from build123d import *

# Parameters (mm, degrees)
F0_W         = 126
F0_H         = 10
F0_R         = 1.5
F1_DEPTH     = 8
F2_T1_DEPTH  = 4
F2_T3_DEPTH  = 18
F2_T5_DEPTH  = 129
F2_T7_DEPTH  = 13
F2_S11_W     = 2
F2_S11_H     = 2
F2_T12_DEPTH = 2
F2_S17_W     = 2
F2_S17_H     = 2
F2_T18_DEPTH = 2
F3_T1_DEPTH  = 11
F3_T3_DEPTH  = 4
F3_T5_DEPTH  = 127
F3_S9_W      = 2.04
F3_S9_H      = 2.04
F3_T10_DEPTH = 2.04
F3_S15_W     = 2.04
F3_S15_H     = 2.04
F3_T16_DEPTH = 2.04


# Not quite as in the source:
# - a fillet or chamfer that OpenCascade refuses, or shapes differently, is made with other operations: its cross-section is extruded or revolved along the edge and cut away or added


with BuildPart() as f1:
    # F0 (on Front) → F1 (new body)
    with BuildSketch(Plane.XZ):
        with Locations((0, 5)):
            Rectangle(F0_W, F0_H)
        with Locations((-60, 5)):
            Circle(F0_R, mode=Mode.SUBTRACT)
        with Locations((-40, 5)):
            Circle(F0_R, mode=Mode.SUBTRACT)
        with Locations((60, 5)):
            Circle(F0_R, mode=Mode.SUBTRACT)
    extrude(amount=F1_DEPTH)

    # F2: fillet of radius 2 on 7 edges, made by hand

    # F2_s2 → F2_t1 (cut)
    with BuildSketch(Plane.XZ.offset(2)):
        with BuildLine():
            ThreePointArc((63, 8), (62.4142135624, 9.4142135624), (61, 10))
            Line((61, 10), (63, 10))
            Line((63, 10), (63, 8))
        make_face()
    extrude(amount=F2_T1_DEPTH, mode=Mode.SUBTRACT)

    # F2_s4 → F2_t3 (cut)
    with BuildSketch(Plane.XZ.offset(-5)):
        with BuildLine():
            ThreePointArc((-63, 8), (-62.4142135624, 9.4142135624), (-61, 10))
            Line((-61, 10), (-63, 10))
            Line((-63, 10), (-63, 8))
        make_face()
        with BuildLine():
            ThreePointArc((61, 0), (62.4142135624, 0.5857864376), (63, 2))
            Line((63, 2), (63, 0))
            Line((63, 0), (61, 0))
        make_face()
    extrude(amount=F2_T3_DEPTH, mode=Mode.SUBTRACT)

    # F2_s6 → F2_t5 (cut)
    with BuildSketch(Plane.YZ.offset(-68)):
        with BuildLine():
            ThreePointArc((-2, 10), (-0.5857864376, 9.4142135624), (0, 8))
            Line((0, 8), (0, 10))
            Line((0, 10), (-2, 10))
        make_face()
        with BuildLine():
            ThreePointArc((-6, 10), (-7.4142135624, 9.4142135624), (-8, 8))
            Line((-8, 8), (-8, 10))
            Line((-8, 10), (-6, 10))
        make_face()
    extrude(amount=F2_T5_DEPTH, mode=Mode.SUBTRACT)

    # F2_s8 → F2_t7 (cut)
    with BuildSketch(Plane.XY.offset(-5)):
        with BuildLine():
            ThreePointArc((63, -2), (62.4142135624, -0.5857864376), (61, 0))
            Line((61, 0), (63, 0))
            Line((63, 0), (63, -2))
        make_face()
        with BuildLine():
            ThreePointArc((63, -6), (62.4142135624, -7.4142135624), (61, -8))
            Line((61, -8), (63, -8))
            Line((63, -8), (63, -6))
        make_face()
    extrude(amount=F2_T7_DEPTH, mode=Mode.SUBTRACT)


with BuildPart() as f2_tool10:
    # F2_s11 → F2_t12 (new body)
    with BuildSketch(Plane.YZ.offset(61)):
        with Locations((-1, 9)):
            Rectangle(F2_S11_W, F2_S11_H)
    extrude(amount=F2_T12_DEPTH)

    # F2_s13 → F2_t14 (revolve, cut)
    with BuildSketch(Plane(origin=(61, -2, 8), x_dir=(0, -0.7071067812, -0.7071067812), z_dir=(0, -0.7071067812, 0.7071067812))):
        with BuildLine():
            ThreePointArc((0, -2), (2, 0), (0, 2))
            Line((0, 2), (0, -2))
        make_face()
    revolve(axis=Axis((61, -2, 8), (1, 0, 0)), mode=Mode.SUBTRACT)


with BuildPart() as f1_1:
    add(f1.part)

    # F2_t9: cut F2_tool10
    add(f2_tool10.part, mode=Mode.SUBTRACT)


with BuildPart() as f2_tool16:
    # F2_s17 → F2_t18 (new body)
    with BuildSketch(Plane.XZ.offset(6)):
        with Locations((62, 9)):
            Rectangle(F2_S17_W, F2_S17_H)
    extrude(amount=F2_T18_DEPTH)

    # F2_s19 → F2_t20 (revolve, cut)
    with BuildSketch(Plane(origin=(61, -6, 8), x_dir=(-0.7071067812, 0, -0.7071067812), z_dir=(-0.7071067812, 0, 0.7071067812))):
        with BuildLine():
            ThreePointArc((0, -2), (2, 0), (0, 2))
            Line((0, 2), (0, -2))
        make_face()
    revolve(axis=Axis((61, -6, 8), (0, -1, 0)), mode=Mode.SUBTRACT)


with BuildPart() as f1_2:
    add(f1_1.part)

    # F2_t15: cut F2_tool16
    add(f2_tool16.part, mode=Mode.SUBTRACT)

    # F3: fillet of radius 2 on 7 edges, made by hand

    # F3_s2 → F3_t1 (cut)
    with BuildSketch(Plane.XY.offset(2)):
        with BuildLine():
            ThreePointArc((-63, -2), (-62.4142135624, -0.5857864376), (-61, 0))
            Line((-61, 0), (-63, 0))
            Line((-63, 0), (-63, -2))
        make_face()
        with BuildLine():
            ThreePointArc((-63, -6), (-62.4142135624, -7.4142135624), (-61, -8))
            Line((-61, -8), (-63, -8))
            Line((-63, -8), (-63, -6))
        make_face()
    extrude(amount=F3_T1_DEPTH, mode=Mode.SUBTRACT)

    # F3_s4 → F3_t3 (cut)
    with BuildSketch(Plane.XZ.offset(2)):
        with BuildLine():
            ThreePointArc((-63, 2), (-62.4142135624, 0.5857864376), (-61, 0))
            Line((-61, 0), (-63, 0))
            Line((-63, 0), (-63, 2))
        make_face()
    extrude(amount=F3_T3_DEPTH, mode=Mode.SUBTRACT)

    # F3_s6 → F3_t5 (cut)
    with BuildSketch(Plane.YZ.offset(-61)):
        with BuildLine():
            ThreePointArc((0, 2), (-0.5857864376, 0.5857864376), (-2, 0))
            Line((-2, 0), (0, 0))
            Line((0, 0), (0, 2))
        make_face()
        with BuildLine():
            ThreePointArc((-6, 0), (-7.4142135624, 0.5857864376), (-8, 2))
            Line((-8, 2), (-8, 0))
            Line((-8, 0), (-6, 0))
        make_face()
    extrude(amount=F3_T5_DEPTH, mode=Mode.SUBTRACT)


with BuildPart() as f3_tool8:
    # F3_s9 → F3_t10 (new body)
    with BuildSketch(Plane.YZ.offset(-61)):
        with Locations((-0.98, 0.98)):
            Rectangle(F3_S9_W, F3_S9_H)
    extrude(amount=-F3_T10_DEPTH)

    # F3_s11 → F3_t12 (revolve, cut)
    with BuildSketch(Plane(origin=(-61, -2, 2), x_dir=(0, -0.7071067812, 0.7071067812), z_dir=(0, -0.7071067812, -0.7071067812))):
        with BuildLine():
            ThreePointArc((0, -2), (2, 0), (0, 2))
            Line((0, 2), (0, -2))
        make_face()
    revolve(axis=Axis((-61, -2, 2), (-1, 0, 0)), mode=Mode.SUBTRACT)


with BuildPart() as f1_3:
    add(f1_2.part)

    # F3_t7: cut F3_tool8
    add(f3_tool8.part, mode=Mode.SUBTRACT)


with BuildPart() as f3_tool14:
    # F3_s15 → F3_t16 (new body)
    with BuildSketch(Plane.YZ.offset(-61)):
        with Locations((-7.02, 0.98)):
            Rectangle(F3_S15_W, F3_S15_H)
    extrude(amount=-F3_T16_DEPTH)

    # F3_s17 → F3_t18 (revolve, cut)
    with BuildSketch(Plane(origin=(-61, -6, 2), x_dir=(0, 0.7071067812, 0.7071067812), z_dir=(0, -0.7071067812, 0.7071067812))):
        with BuildLine():
            ThreePointArc((0, -2), (2, 0), (0, 2))
            Line((0, 2), (0, -2))
        make_face()
    revolve(axis=Axis((-61, -6, 2), (-1, 0, 0)), mode=Mode.SUBTRACT)


with BuildPart() as f1_4:
    add(f1_3.part)

    # F3_t13: cut F3_tool14
    add(f3_tool14.part, mode=Mode.SUBTRACT)


solid = f1_4.part
The model under review builds one solid part; all positions refer to its coordinate system, in mm. Round coordinates to 2 decimals unless told otherwise and drop trailing zeros. Loops run counter-clockwise (first coordinate to the right, second up) from the corner with the lowest first, then second, coordinate; pieces in that order, holes last. Notation, with made-up numbers: M 89.25,16.5 L 102.25,16.5 A18 cw 102.25,42.5 Z; hole C 19.5,-19 d5. An arc over 180 degrees is marked long. Answer as a JSON object with one key per item and string values.
Item 1: The part is to be moulded in two halves that separate along X. For faces 1 (the face through (-1, 0, 5)), 2 (the face through (-41.5, -3.94, 5.07)), 3 (the face through (62.4, -3.95, 0.57)), say which applies: +X half, -X half, draft (parallel to the pull), parting line (faces both ways), or undercut.
Check sheet entries:
{"face 1": "draft", "face 2": "undercut", "face 3": "+X half"}
Item 2: For line 1 along Z through (x, y) = (60, -4); line 2 along X through (y, z) = (-0.25, 5.75); line 3 along Z through (x, y) = (-6.5, -1.75), list the stretches that pass through material, from the lowest coordinate up.
Check sheet entries:
{"line 1": "0 to 3.5, 6.5 to 10", "line 2": "-61.97 to -61.3, -58.7 to -41.3, -38.7 to 58.7, 61.3 to 61.97", "line 3": "0.02 to 9.98"}
Item 3: We need section D-D, the plane z = 5. State the section outline as (x, y) points, and give its area (3 significant figures).
Check sheet entries:
{"outline": "M -63,-6 A2 ccw -61.5,-7.94 L -61.5,-0.06 A2 ccw -63,-2 Z; M -58.5,-8 L -41.5,-8 L -41.5,0 L -58.5,0 Z; M -38.5,-8 L 58.5,-8 L 58.5,0 L -38.5,0 Z; M 61.5,-7.94 A2 ccw 63,-6 L 63,-2 A2 ccw 61.5,-0.06 Z", "area": "933 mm2"}
Item 4: We need section B-B, the plane y = -4.75. State the section outline as (x, z) points.
Check sheet entries:
{"outline": "M -63,2 A2 ccw -61,0 L 61,0 A2 ccw 63,2 L 63,8 A2 ccw 61,10 L -61,10 A2 ccw -63,8 Z; hole C -60,5 d3; hole C -40,5 d3; hole C 60,5 d3"}
Item 5: We need section C-C, the plane x = 25. State the section outline as (y, z) points.
Check sheet entries:
{"outline": "M -8,2 A2 ccw -6,0 L -2,0 A2 ccw 0,2 L 0,8 A2 ccw -2,10 L -6,10 A2 ccw -8,8 Z"}
Item 6: We need section A-A, the plane x = -40. State the section outline as (y, z) points.
Check sheet entries:
{"outline": "M -8,2 A2 ccw -6,0 L -2,0 A2 ccw 0,2 L 0,3.5 L -8,3.5 Z; M -8,6.5 L 0,6.5 L 0,8 A2 ccw -2,10 L -6,10 A2 ccw -8,8 Z"}
